Drawing for the job (mm, zero at the part's lowest x, y, z). Round coordinates to 2 decimals unless told otherwise and drop trailing zeros. Order: outer loops, then holes, each group sorted by start corner. A loop starts at its lowest first (then second) coordinate and runs counter-clockwise, first axis right, second up. Notation, with made-up numbers: (37.5, 7) - (79.5, 7) arc R5 ccw to (79.5, 11) - close; hole circle Ø4 at (51, 84). An arc over 180 degrees is marked (long way). Put each result on its own line as item: value. Start each with the question number.
Item 1: Pin check, flat tips, straight feed: pin 1 Ø1.5 at (y, z) = (1, 30) entering from -X; pin 2 Ø0.9 at (y, z) = (1, 46) entering from +X. Stop position of each tip, or through.
Item 2: Saw through at A-A on x = 85.5. List the corners of the cut face in (y, z), plus the area to 3 significant figures.
Item 3: Saw through at C-C on z = 39. List the corners of the cut face in (x, y) (1 decimal).
Item 4: Saw through at B-B on y = 2. State how many separate pieces and enclosed holes the cut face has, plus the area to 3 significant figures.
Item 5: Probe probe 1 along Z at (x, y) = (77, 2.4); probe 2 along X at (y, z) = (1.75, 62.5) (1 decimal); probe 3 along X at (y, z) = (2.3, 58) (1 decimal). List the from-to ranges inside material, lowest first.
Item 6: Saw through at D-D on z = 52.5. List the corners of the cut face in (x, y) (1 decimal).
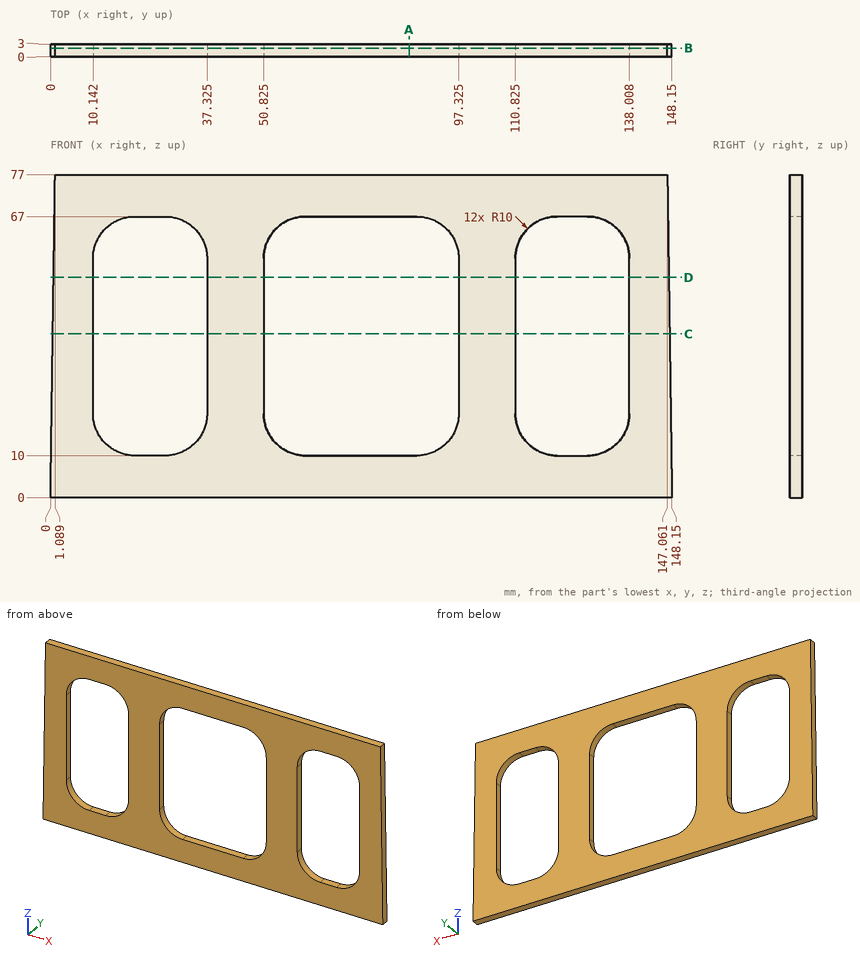
Results found:
1. pin 1: stops at x = 0.41
1. pin 2: stops at x = 147.51
2. outline: (0, 0) - (3, 0) - (3, 10) - (0, 10) - close; (0, 67) - (3, 67) - (3, 77) - (0, 77) - close
2. area: 60.0 mm²
3. outline: (0.6, 0) - (10.1, 0) - (10.1, 3) - (0.6, 3) - close; (37.3, 0) - (50.8, 0) - (50.8, 3) - (37.3, 3) - close; (97.3, 0) - (110.8, 0) - (110.8, 3) - (97.3, 3) - close; (138, 0) - (147.6, 0) - (147.6, 3) - (138, 3) - close
4. separate pieces: 1
4. enclosed holes: 3
4. area: 5,830 mm²
5. probe 1: z = 0 to 10, 67 to 77
5. probe 2: x = 0.9 to 11.8, 35.7 to 52.5, 95.7 to 112.5, 136.4 to 147.3
5. probe 3: x = 0.8 to 10.2, 37.3 to 50.9, 97.3 to 110.9, 138 to 147.3
6. outline: (0.7, 0) - (10.1, 0) - (10.1, 3) - (0.7, 3) - close; (37.3, 0) - (50.8, 0) - (50.8, 3) - (37.3, 3) - close; (97.3, 0) - (110.8, 0) - (110.8, 3) - (97.3, 3) - close; (138, 0) - (147.4, 0) - (147.4, 3) - (138, 3) - close
